Here's the drawing with two shaded views (mm, measured from the low corner). I have some questions. Round coordinates to 2 decimals unless told otherwise and drop trailing zeros. Loops run counter-clockwise (first coordinate to the right, second up) from the corner with the lowest first, then second, coordinate; pieces in that order, holes last.
(1) Thinking about a two-plate mould opening in X: for the marked faces 1, 2, 3 and 4, which applies, released by +X, released by -X, zero draft, split by the parting line, or undercut?
(2) I want a section at A-A on z = 20.5. Write out the boundary of the cut face in (x, y), plus the area to 3 significant figures.
(3) I want a section at B-B on y = 20.5. Write out the boundary of the cut face in (x, z).
(4) I want a section at C-C on x = 18.75. Write out the boundary of the cut face in (y, z).
(5) I want a section at D-D on z = 29.5. Write out the boundary of the cut face in (x, y), plus the area to 3 significant figures.
(6) Will these pins go through, and if not, where does the flat tip stop? pin 1 Ø5 at (x, y) = (2, 20.5) entering from +Z; pin 2 Ø20.5 at (y, z) = (13, 23.5) entering from +X; pin 3 Ø6 at (x, z) = (17.5, 5.5) entering from -Y; pin 4 Ø10 at (y, z) = (20.5, 7.5) entering from -X.
(7) If I drill on line 1 along X through (y, z) = (4, 29); line 2 along X through (y, z) = (32, 8); line 3 along Y through (x, z) = (11.5, 21), over which ranges is the centre line in solid material (lowest first)?
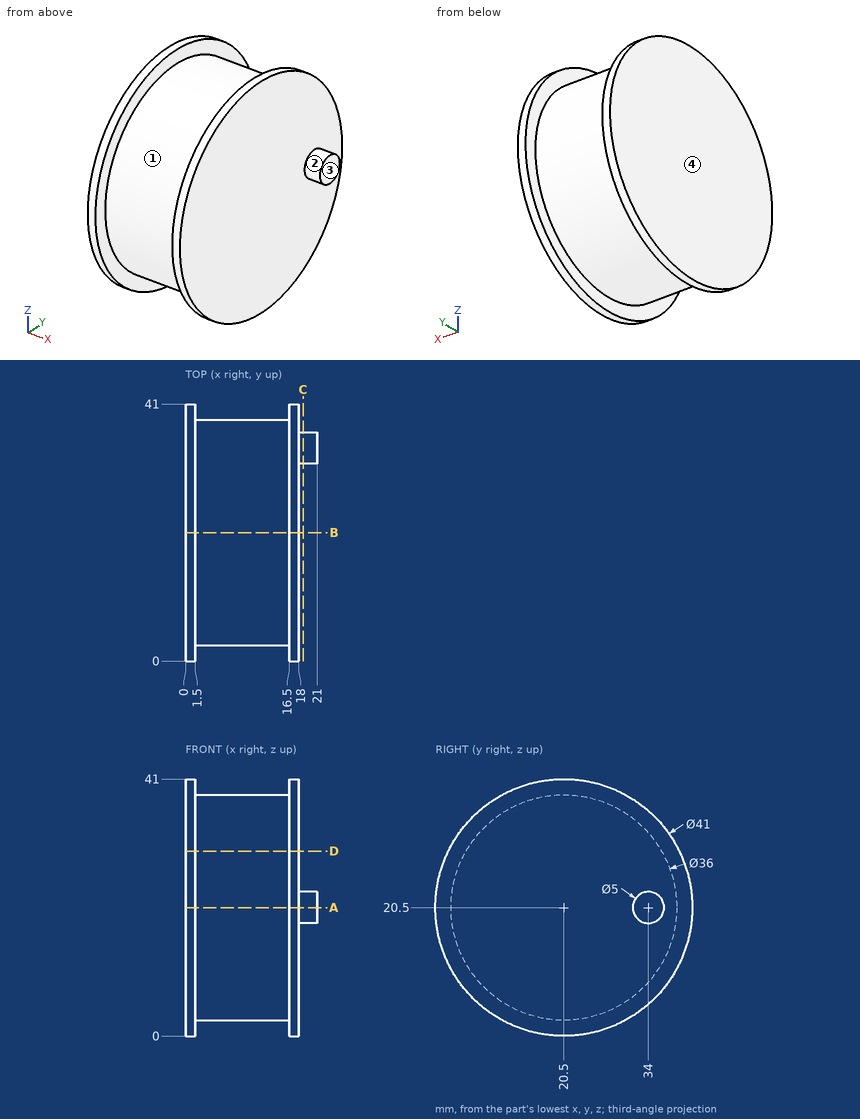
Filled sheet:
1. face 1: undercut
1. face 2: zero draft
1. face 3: released by +X
1. face 4: released by -X
2. outline: (0, 0) - (1.5, 0) - (1.5, 2.5) - (16.5, 2.5) - (16.5, 0) - (18, 0) - (18, 31.5) - (21, 31.5) - (21, 36.5) - (18, 36.5) - (18, 41) - (16.5, 41) - (16.5, 38.5) - (1.5, 38.5) - (1.5, 41) - (0, 41) - close
2. area: 678 mm2
3. outline: (0, 0) - (1.5, 0) - (1.5, 2.5) - (16.5, 2.5) - (16.5, 0) - (18, 0) - (18, 41) - (16.5, 41) - (16.5, 38.5) - (1.5, 38.5) - (1.5, 41) - (0, 41) - close
4. outline: circle Ø5 at (34, 20.5)
5. outline: (0, 2.08) - (1.5, 2.08) - (1.5, 4.91) - (16.5, 4.91) - (16.5, 2.08) - (18, 2.08) - (18, 38.92) - (16.5, 38.92) - (16.5, 36.09) - (1.5, 36.09) - (1.5, 38.92) - (0, 38.92) - close
5. area: 578 mm2
6. pin 1: stops at z = 41
6. pin 2: stops at x = 18
6. pin 3: stops at y = 3.88
6. pin 4: stops at x = 0
7. line 1: x = 0 to 1.5, 16.5 to 18
7. line 2: x = 0 to 18
7. line 3: y = 2.51 to 38.49
